Input: part model. Units: mm. Frame: model coordinates. A direction names the side the tool comes from. Coordinates: 2 decimals unless noted, no trailing zeros. Loops run counter-clockwise (first coordinate to the right, second up) from the corner with the lowest first, then second, coordinate; pieces in that order, holes last.
(1) Section B-B, the plane z = -50. Return loops of the section in (x, y) (1 decimal).
(2) Section A-A, the plane x = 10. Return loops of the section in (y, z).
(3) Contact query for flat-ended pins moving along their axis: P1, Ø10, axis at x = 10.01, z = -45.52, coming from the +Y side; P2, Ø12, axis at x = 63, y = 52, coming from the +Z side; P3, Ø10, axis at x = 20, y = 32.5, coming from the +Z side; P4, Ø8, axis at x = 11.5, y = 17.5, coming from the +Z side. Output: stop coordinate, or through.
(4) Section D-D, the plane y = 52. Return loops of the section in (x, z).
(5) Section C-C, the plane y = 35. Give the number of separate pieces and of enclosed holes in the cut face, then the cut area to 3 significant figures.
(6) Mould query, pull axis X, two halves, no side actions, for faces 3 (the face through (35.304, 8.482, -18.29)), 4 (the face through (37, 49, -58.014)), 5 (the face through (57.743, 22.789, -31.344)), 6 (the face through (0, 22, -35)). Classes: released by +X, released by -X, zero draft, split by the parting line, or undercut.
(7) Line query: L1, parallel to X at y = 44.5, z = -47; L2, parallel to Z at x = 64.5, y = 3; L3, parallel to X at y = 16, z = -49.5. Output: solid intervals per line, ascending.
(8) Set-up query: faces 1 (the face through (61.625, 28.601, -48.863)), 2 (the face through (54.2, 37.8, -33.02)). Return all of +Z, -Z, +X, -X, +Y, -Y with unobstructed straight access to the full face (end or side cutting, diameter ignored); none if empty.
```python
from build123d import *

# Parameters (mm, degrees)
SKETCH1_W          = 75.9968
SKETCH1_H          = 58.0136
SKETCH1_R          = 18.2625
EXTRUDE1_DEPTH     = 58.0136
CUT_EXTRUDE1_DEPTH = 76.9968
SKETCH3_R          = 20.701
CUT_EXTRUDE2_DEPTH = 33.02
FILLET1_R          = 0.762
HOLE1_D            = 10.9982
HOLE1_DEPTH        = 58.0136


with BuildPart() as part:
    # Sketch1 → Extrude1 (new body)
    with BuildSketch(Plane.XY):
        with Locations((37.9984, 29.0068)):
            Rectangle(SKETCH1_W, SKETCH1_H)
        with Locations((37.9984, 29.0068)):
            Circle(SKETCH1_R, mode=Mode.SUBTRACT)
    extrude(amount=-EXTRUDE1_DEPTH)

    # Sketch2 → Cut-Extrude1 (cut, through all)
    with BuildSketch(Plane(origin=(75.9968, 0, 0), x_dir=(0, 0, -1), z_dir=(1, 0, 0))):
        Polygon((0, 58.0136), (33.02, 58.0136), (0, 6.5024), align=None)
    extrude(amount=-CUT_EXTRUDE1_DEPTH, mode=Mode.SUBTRACT)

    # Sketch3 → Cut-Extrude2 (cut)
    with BuildSketch(Plane(origin=(0, 0, 0), x_dir=(-1, 0, 0), z_dir=(0, 0, -1))):
        with Locations(Location((-37.9984, 29.0068, 0), (0, 0, 180))):  # turned: the seam where the file's is
            Circle(SKETCH3_R)
    extrude(amount=CUT_EXTRUDE2_DEPTH, mode=Mode.SUBTRACT)

    # Fillet1
    fillet1_edges = [part.edges().sort_by_distance(p)[0] for p in [
        (17.2974, 29.0068, -33.02),
    ]]
    fillet(fillet1_edges, radius=FILLET1_R)

    # Hole1
    with Locations(Plane(origin=(0, 58.0136, 0), x_dir=(-1, 0, 0), z_dir=(0, 1, 0))):
        with Locations((-10.0076, -45.5168), (-65.9892, -45.5168)):
            Hole(HOLE1_D / 2, depth=HOLE1_DEPTH)

    # Sketch6 → Cut-Revolve1 (revolve, cut)
    with BuildSketch(Plane(origin=(0, 29.0068, 0), x_dir=(-1, 0, 0), z_dir=(0, 1, 0)), mode=Mode.PRIVATE) as cut_revolve1_sk:
        Polygon((-17.2974, -29.6926), (-17.2974, -30.4546), (-16.9164, -30.0736), align=None)
        Polygon((-19.7359, -56.8451), (-19.7359, -58.0136), (-18.5674, -58.0136), align=None)
    revolve(cut_revolve1_sk.sketch.rotate(Axis((37.9984, 29.0068, 17.508123997), (0, 0, -1)), 180), axis=Axis((37.9984, 29.0068, 17.508123997), (0, 0, -1)), mode=Mode.SUBTRACT)  # turned: the seam where the file's is


solid = part.part
```
Report:
1. outline: (0, 0) - (6.8, 0) - (6.8, 58) - (0, 58) - close; (13.2, 0) - (62.8, 0) - (62.8, 58) - (13.2, 58) - close; (69.2, 0) - (76, 0) - (76, 58) - (69.2, 58) - close; hole circle Ø36.5 at (38, 29)
2. outline: (0, -58.01) - (58.01, -58.01) - (58.01, -51.02) - (0, -51.02) - close; (0, -40.02) - (58.01, -40.02) - (58.01, -33.02) - (6.5, 0) - (0, 0) - close
3. P1: passes through
3. P2: stops at z = -25.32
3. P3: stops at z = -13.96
3. P4: stops at z = -4.49
4. outline: (0, -58.01) - (76, -58.01) - (76, -29.17) - (0, -29.17) - close; hole circle Ø11 at (10.01, -45.52); hole circle Ø11 at (65.99, -45.52)
5. separate pieces: 2
5. enclosed holes: 2
5. area: 1,380 mm2
6. face 3: undercut
6. face 4: zero draft
6. face 5: undercut
6. face 6: released by -X
7. L1: x = 0 to 4.71, 15.3 to 28.33, 47.67 to 60.69, 71.28 to 76
7. L2: z = -58.01 to -50.81, -40.22 to 0
7. L3: x = 0 to 6.22, 13.8 to 25.18, 50.82 to 62.2, 69.78 to 76
8. face 1: +Y, -Y
8. face 2: +Z
